Build history of the part. All positions in model axes, mm. A direction names the side the tool comes from. Give positions to 0.01 mm unless a question says otherwise; leave off trailing zeros. Order: outer loops, then holes, each group sorted by start corner. A loop starts at its lowest first (then second) coordinate and runs counter-clockwise, first axis right, second up. Notation, with made-up numbers: (-25.5, 45.25) - (-18.5, 45.25) arc R14 ccw to (-18.5, 67.25) - close; hole circle Ø1 at (-9, 83). An arc over 180 degrees is marked (long way). Answer in a Markdown table with one row per item.
Autodesk Inventor part; units mm, degrees
ref_plane "YZ Plane" through (0, 0, 0) normal (1, 0, 0) x (0, 1, 0)
ref_plane "XZ Plane" through (0, 0, 0) normal (0, 1, 0) x (-1, 0, 0)
ref_plane "XY Plane" through (0, 0, 0) normal (0, 0, 1) x (1, 0, 0)
sketch "Sketch1" plane through (0, 0, 0) normal (0, 0, 1) x (1, 0, 0)
  circle A0 centre (0, 0) radius 10
  dimension "d0" = 20
sketch "Sketch2" plane through (0, 0, 0) normal (1, 0, 0) x (0, 1, 0)
  line L0 (0, 0) -> (0, -150)
  line L1 (10, -160) -> (200, -160)
  arc A0 (0, -150) -> (10, -160) centre (10, -150) ccw
  point P0 (0, -160)
  dimension "d1" = 160
  dimension "d2" = 200
  dimension "d3" = 10
sweep "Sweep1" add profiles "Sketch1" path "Sketch2"
thread "Thread1"
sketch "Sketch3" plane through (0, 0, 0) normal (0, 1, 0) x (-1, 0, 0)
  circle A0 centre (0, 0) radius 17.5
  dimension "d8" = 35
extrude "Extrusion1" add sketch "Sketch3" along normal blind 20
sketch "Sketch4" plane through (0, 20, 0) normal (0, 1, 0) x (1, 0, 0)
  circle A0 centre (0, 0) radius 10
  dimension "d11" = 20
extrude "Extrusion2" cut sketch "Sketch4" against normal through all
sketch "Sketch5" plane through (0, 0, 0) normal (0, -1, 0) x (1, 0, 0)
  arc A0 (10, -14.3614) -> (-10, -14.3614) centre (0, 0) ccw
  circle A1 centre (0, 0) radius 17.5
  point P0 (-10, -14.3614)
extrude "Extrusion3" cut sketch "Sketch5" along normal blind 10
1. Drop flat-ended pins along their axis: P1, Ø2, axis at x = -7, y = 116, coming from the -Z side; P2, Ø3, axis at y = 29.5, z = -150.5, coming from the -X side; P3, Ø6, axis at x = -7, y = 94.5, coming from the +Z side. Give the stop position or say it passes through.
Check result:
| item | result |
|---|---|
| P1 | stops at z = -168 |
| P2 | stops at x = -6 |
| P3 | stops at z = -150.83 |
2. Cut at A-A on z = 0. Write the cut outline in (x, y), and give its area (3 significant figures).
Check result:
| item | result |
|---|---|
| outline | (-17.5, 0) - (-10, 0) - (-10, 20) - (-17.5, 20) - close; (10, 0) - (17.5, 0) - (17.5, 20) - (10, 20) - close |
| area | 300 mm² |
3. Which spindle directions (+Z, -Z, +X, -X, +Y, -Y) get a long thin tool onto all of the face, cutting with end or side? Do faces 4 (the face through (0, 200, -160)), 5 (the face through (0.1, -3.8, -17.5)), 6 (the face through (-2.17, 106.33, -150.24)). Say none if no direction does.
Check result:
| item | result |
|---|---|
| face 4 | +Z, -Z, +X, -X, +Y |
| face 5 | +Z, -Y |
| face 6 | +Y |
4. Cut at D-D on x = 14. Write the cut outline in (y, z).
Check result:
| item | result |
|---|---|
| outline | (0, -10.5) - (20, -10.5) - (20, 10.5) - (0, 10.5) - close |
5. Two-plate mould, pull along X, no slides. Class faces 1 (the face through (-2.17, 9.76, -83.13)), 2 (the face through (-8, 20, -8)), 3 (the face through (-2.17, 10.14, 9.76)): +X half, -X half, draft (parallel to the pull), parting line (faces both ways), or undercut.
Check result:
| item | result |
|---|---|
| face 1 | parting line |
| face 2 | draft |
| face 3 | undercut |
6. Cut at B-B on y = 139.5. Write the cut outline in (x, z).
Check result:
| item | result |
|---|---|
| outline | circle Ø20 at (0, -160) |
7. Probe line 1 (Z direction, x = 0, y = 15.25); line 2 (X direction, y = 10, z = 0); line 3 (Z direction, x = 0, y = 9). List the from-to ranges inside material, lowest first.
Check result:
| item | result |
|---|---|
| line 1 | z = -170 to -150, -17.5 to -10, 10 to 17.5 |
| line 2 | x = -17.5 to -10, 10 to 17.5 |
| line 3 | z = -169.97 to -10, 10 to 17.5 |
8. Cut at C-C on z = -144. Write the cut outline in (x, y).
Check result:
| item | result |
|---|---|
| outline | circle Ø20 at (0, 0) |
